Build history of the part. All positions in model axes, mm. Face numbers are marked on the shaded views. A direction names the side the tool comes from. Give positions to 0.01 mm unless a question says otherwise; leave off trailing zeros. Order: outer loops, then holes, each group sorted by start corner. A loop starts at its lowest first (then second) coordinate and runs counter-clockwise, first axis right, second up. Notation, with made-up numbers: (13, 9) - (43, 9) arc R14 cw to (43, 30) - close; hole circle Ø5 at (17, 49). An arc over 180 degrees is marked (long way). Write each question's results on one line, items separated by ' | '. Start each with the question number.
1) Cut at B-B on x = -4. List the corners of the cut face in (y, z).
2) Cut at C-C on z = 0.75. List the corners of the cut face in (x, y), plus the area to 3 significant figures.
3) Tool access for the marked faces 1 and 2: list every direction of +Z, -Z, +X, -X, +Y, -Y with a clear straight run to the whole face (end or side of a thin tool).
4) Drop flat-ended pins along their axis: pin 1 Ø1.5 at (x, y) = (-4, -4.5) entering from +Z; pin 2 Ø0.8 at (y, z) = (4.5, 1.5) entering from -X. Give the stop position or say it passes through.
5) Drill centre lines: line 1 along Z through (x, y) = (-4.5, -0.25); line 2 along X through (y, z) = (0.25, 0.5); line 3 along Z through (x, y) = (0.5, 8.75). Where is each one in solid material? Low to high. Write a range as from..to.
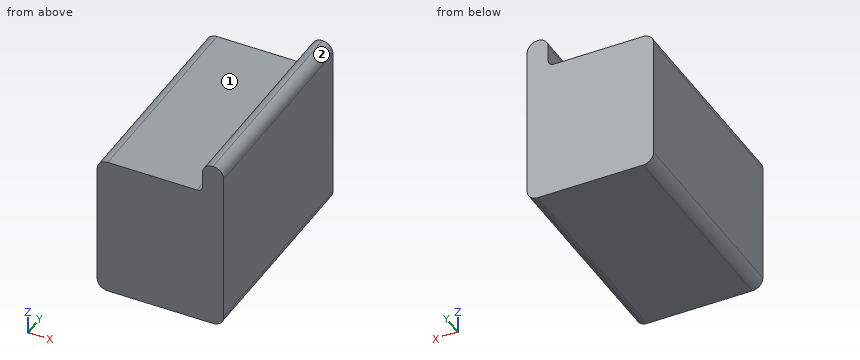
Autodesk Fusion 360 part; units mm, degrees
sketch "Sketch1" plane through (0, 0, 0) normal (0, 1, 0) x (1, 0, 0)
  line L0 (0, 0) -> (0, -3)
  line L1 (0, -3) -> (2, -3)
  line L2 (2, -3) -> (2, 13.5)
  line L3 (2, 13.5) -> (-10, 13.5)
  line L4 (-10, 13.5) -> (-10, 0)
  line L5 (-10, 0) -> (0, 0)
  dimension "d1" = 3
  dimension "d2" = 10
  dimension "d4" = 13.5
  dimension "d5" = 2
extrude "Extrude1" add sketch "Sketch1" along normal mid plane 20
fillet "Fillet1" radius 1 5 edges at (2, 0, -13.5) (-10, 0, -13.5) (-10, 0, 0) (2, 0, 3) (0, 0, 3)
fillet "Fillet2" radius 0.5 1 edges at (0, 0, 0)
Results:
1) outline: (-10, -13.5) - (10, -13.5) - (10, 0) - (-10, 0) - close
2) outline: (0, -10) - (2, -10) - (2, 10) - (0, 10) - close | area: 40.0 mm^2
3) face 1: +Z, -X, +Y, -Y | face 2: +Z, +X, +Y, -Y
4) pin 1: z = 0 | pin 2: x = 0
5) line 1: -13.5..0 | line 2: 0..2 | line 3: -13.5..2.87
